Check sheet for the modelled part. Datum: model origin and axes. Units: mm. Give positions to 0.01 mm unless a question says otherwise; leave off trailing zeros. Loops run counter-clockwise (first coordinate to the right, second up) from the corner with the lowest first, then second, coordinate; pieces in that order, holes last. Notation, with made-up numbers: (75.25, 7.5) -> (118.25, 7.5) arc R29 cw to (118.25, 46.5) -> close; hole circle Ø5 at (-15, 54). An arc over 180 degrees is marked (long way). Write each question's results on one line, items separated by ' | '. Start each with the question number.
1. Cross-section at B-B on z = 10. Record the boundary of the cut face in (x, y).
2. Cross-section at A-A on x = -28.5. Record the boundary of the cut face in (y, z).
3. Mould release check, pull along Z, two halves, no side actions. Record for faces 1 (the face through (-34.85, 163.39, 34.31)), 2 (the face through (30.911, 150.266, 40.313)), 3 (the face through (45, 0, -15)): +Z half, -Z half, draft (parallel to the pull), parting line (faces both ways), or undercut.
4. Gauge pin test, flat ends, axial feed: pin 1 Ø8 at (y, z) = (79.5, -9) entering from +X; pin 2 Ø5 at (x, y) = (29.5, 156.5) entering from -Z; pin 3 Ø1 at (y, z) = (34.5, 30) entering from -X. Record the tip position at first contact, or that the pin passes through.
5. Cross-section at C-C on y = 48.5. Record the boundary of the cut face in (x, z), and give its area (3 significant figures).
6. Material ranges on L1, parallel to Z at x = 0, y = 223; L2, parallel to Y at x = 0, z = 48; L3, parallel to Z at x = 5, y = 222, recorded low to high. Write a range as from..to.
from build123d import *

# Parameters (mm, degrees)
SKETCH2_R                 = 50.8
SKETCH2_R_2               = 46.99
COUPLER_EXTRUSION_DEPTH   = 304.8
BULKHEAD_HOLES_REACH      = 327.279
BULKHEAD_HOLES_END_RADIUS = 46.99
SKETCH3_R                 = 1.7526
CIRPATTERN1_COUNT         = 8


with BuildPart() as part:
    # Sketch2 → Coupler Extrusion (new body)
    with BuildSketch(Plane(origin=(0, 0, 0), x_dir=(1, 0, 0), z_dir=(0, 1, 0))):
        with Locations(Location((0, 0, 0), (0, 0, 90))):
            Circle(SKETCH2_R)
        with Locations(Location((0, 0, 0), (0, 0, 90))):
            Circle(SKETCH2_R_2, mode=Mode.SUBTRACT)
    extrude(amount=COUPLER_EXTRUSION_DEPTH)

    # Bulkhead Holes: up to this cylinder (the profile starts outside it)
    bulkhead_holes_end = Plane(origin=(0, 165.1, 0), z_dir=(0, -1, 0)) * Cylinder(BULKHEAD_HOLES_END_RADIUS, 749.538, mode=Mode.PRIVATE)
    # Sketch3 → Bulkhead Holes (cut, up to the surface)
    with BuildSketch(Plane.XY.offset(50.8), mode=Mode.PRIVATE) as bulkhead_holes_sk1:
        with Locations((0, 165.1)):
            Circle(SKETCH3_R)
    bulkhead_holes_tool1 = extrude(bulkhead_holes_sk1.sketch, amount=-BULKHEAD_HOLES_REACH, mode=Mode.PRIVATE) - bulkhead_holes_end
    bulkhead_holes = bulkhead_holes_tool1.solids().sort_by_distance((0, 165.1, 50.8))[0]
    add(bulkhead_holes, mode=Mode.SUBTRACT)

    # CirPattern1: Bulkhead Holes ×8 about axis
    cirpattern1_axis = Axis((0, 304.8, 0), (0, -1, 0))
    for i in range(1, CIRPATTERN1_COUNT):
        add(bulkhead_holes.rotate(cirpattern1_axis, i * 360 / CIRPATTERN1_COUNT), mode=Mode.SUBTRACT)


solid = part.part
Geometry says:
1) outline: (-49.81, 0) -> (-45.91, 0) -> (-45.91, 304.8) -> (-49.81, 304.8) -> close; (45.91, 0) -> (49.81, 0) -> (49.81, 304.8) -> (45.91, 304.8) -> close
2) outline: (0, -42.05) -> (304.8, -42.05) -> (304.8, -37.36) -> (0, -37.36) -> close; (0, 37.36) -> (304.8, 37.36) -> (304.8, 42.05) -> (0, 42.05) -> close
3) face 1: undercut | face 2: parting line | face 3: draft
4) pin 1: x = 50.55 | pin 2: z = -43.03 | pin 3: x = -41.36
5) outline: circle Ø101.6 at (0, 0); hole circle Ø93.98 at (0, 0) | area: 1,170 mm^2
6) L1: -50.8..-46.99, 46.99..50.8 | L2: 0..163.35, 166.85..304.8 | L3: -50.55..-46.72, 46.72..50.55
